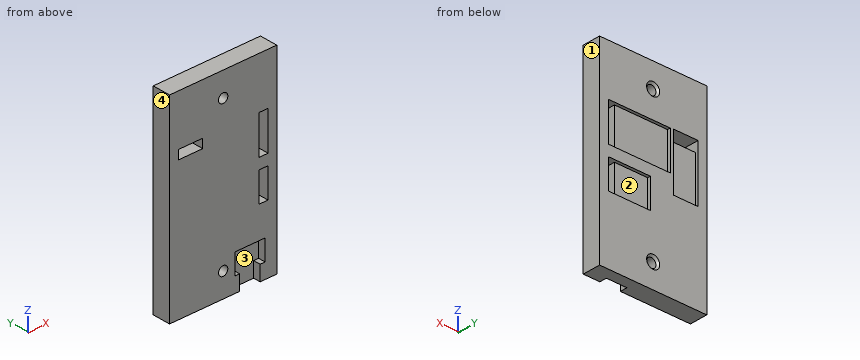
Autodesk Inventor part; units mm, degrees
ref_plane "작업 평면1" through (0, 10, 0) normal (0, 1, 0) x (1, 0, 0)
ref_plane "작업 평면2" through (0, 10, 0) normal (0, 1, 0) x (1, 0, 0)
ref_plane "작업 평면3" through (57.9435, 10, -25.2204) normal (0, 0, 1) x (1, 0, 0)
ref_plane "작업 평면1" through (0, 10, 0) normal (0, 1, 0) x (1, 0, 0)
sketch "스케치3" plane through (0, 10, 0) normal (0, 1, 0) x (1, 0, 0)
  line L0 (108.4435, 113.2704) -> (97.4435, 113.2704)
  line L1 (97.4435, 113.2704) -> (97.4435, 121.7204)
  line L2 (97.4435, 121.7204) -> (108.4435, 121.7204)
  line L3 (108.4435, 121.7204) -> (108.4435, 113.2704)
  line L4 (117.9435, 121.7204) -> (57.9435, 121.7204)
  line L5 (57.9435, 121.7204) -> (57.9435, 11.7204)
  line L6 (117.9435, 11.7204) -> (117.9435, 121.7204)
  line L7 (57.9435, 11.7204) -> (117.9435, 11.7204)
  line L8 (113.0685, 67.6907) -> (89.4185, 67.6907)
  line L9 (89.4185, 67.6907) -> (89.4185, 84.1907)
  line L10 (89.4185, 84.1907) -> (113.0685, 84.1907)
  line L11 (113.0685, 84.1907) -> (113.0685, 67.6907)
  line L12 (113.0684, 40.1407) -> (108.0685, 40.1407)
  line L13 (108.0685, 67.6907) -> (113.0685, 67.6907)
  line L14 (113.0684, 61.6907) -> (113.0684, 40.1407)
  line L15 (113.0685, 67.6907) -> (108.0685, 67.6907)
  line L16 (108.0685, 67.6907) -> (108.0685, 84.1907)
  line L17 (108.0685, 84.1907) -> (113.0685, 84.1907)
  line L18 (113.0685, 84.1907) -> (113.0685, 67.6907)
  line L19 (76.5185, 39.8907) -> (62.8185, 39.8907)
  line L20 (62.8185, 39.8907) -> (62.8185, 44.8907)
  line L21 (62.8185, 44.8907) -> (76.5185, 44.8907)
  line L22 (76.5185, 44.8907) -> (76.5185, 39.8907)
  line L23 (113.0684, 61.6907) -> (78.3675, 61.6907)
  circle A0 centre (87.9435, 25.2204) radius 2.6
  circle A1 centre (87.9435, 108.2204) radius 2.6
  line L24 (78.3675, 40.1407) -> (113.0684, 40.1407)
  line L25 (78.3675, 40.1407) -> (78.3675, 61.6907)
  line L26 (76.5185, 39.8907) -> (76.5185, 71.6407)
  line L27 (62.8185, 39.8907) -> (62.8185, 71.6407)
  line L28 (76.5185, 71.6407) -> (62.8185, 71.6407)
  line L29 (108.0685, 61.6907) -> (108.0685, 40.1407)
  point P0 (0, 0)
  dimension "d8" = 9.5
  dimension "d46" = 5.2
  dimension "d47" = 5.2
extrude "돌출2" add sketch "스케치3" against normal blind 10 contours L3 L4 L6 L7 L5 L1 L0 | L0 L1 L2 L3 | L8 L16 L10 L11 | L8 L9 L10 L16 | L12 L29 L23 L14 | L24 L25 L23 L29 | L19 L20 L21 L22 | L21 L27 L28 L26 | A0 | A1
sketch "스케치4" plane through (0, 10, 0) normal (0, 1, 0) x (1, 0, 0)
  point P0 (0, 0)
sketch "스케치5" plane through (117.9435, 10, -121.7204) normal (0, 0, -1) x (-1, 0, 0)
  point P0 (117.9435, -10)
extrude "돌출5" cut sketch "스케치3" against normal through all contours L0 L1 L2 L3
sketch "스케치6" plane through (0, 0, 0) normal (0, -1, 0) x (1, 0, 0)
  line L0 (57.9435, -121.7204) -> (97.4435, -121.7204)
  line L1 (97.4435, -121.7204) -> (57.9435, -121.7204)
  line L2 (113.0685, -71.6204) -> (108.0685, -71.6204)
  line L3 (113.0685, -80.2704) -> (113.0685, -71.6204)
  line L4 (78.3685, -80.2704) -> (113.0685, -80.2704)
  line L5 (78.3685, -58.4704) -> (78.3685, -80.2704)
  line L6 (113.0685, -58.4704) -> (78.3685, -58.4704)
  line L7 (113.0685, -67.1204) -> (113.0685, -58.4704)
  line L8 (108.0685, -67.1204) -> (113.0685, -67.1204)
  line L9 (108.0685, -71.6204) -> (108.0685, -67.1204)
  line L10 (117.9435, -121.7204) -> (108.4435, -121.7204)
  line L11 (111.4435, -108.7204) -> (94.443, -108.7204)
  line L12 (111.4435, -108.7204) -> (111.4435, -113.2704)
  line L13 (94.443, -108.7204) -> (94.443, -113.2704)
  line L14 (111.4435, -113.2704) -> (94.443, -113.2704)
  point P0 (0, 0)
sketch "스케치7" plane through (0, 0, 0) normal (0, -1, 0) x (1, 0, 0)
  point P0 (0, 0)
sketch "스케치8" plane through (0, 0, 0) normal (0, -1, 0) x (1, 0, 0)
  point P0 (0, 0)
extrude "돌출6" cut sketch "스케치6" against normal blind 4 contours L12 L14 L13 L11
extrude "돌출7" add sketch "스케치3" against normal blind 6 contours L0 L1 L2 L3
sketch "스케치9" plane through (0, 0, 0) normal (0, -1, 0) x (1, 0, 0)
  line L0 (111.4435, -108.7204) -> (111.4435, -113.2704)
  line L1 (111.4435, -108.7204) -> (111.4435, -101.7204)
  line L2 (111.4435, -101.7204) -> (94.443, -101.7204)
  line L3 (94.443, -113.2704) -> (94.443, -108.7204)
  line L4 (94.443, -101.7204) -> (94.443, -108.7204)
  line L5 (94.443, -108.7204) -> (111.4435, -108.7204)
  line L6 (111.4435, -108.7204) -> (94.443, -108.7204)
  point P0 (0, 0)
  dimension "d25" = 7
extrude "돌출8" cut sketch "스케치9" against normal blind 4
sketch "스케치10" plane through (0, 10, 0) normal (0, 1, 0) x (1, 0, 0)
  circle A0 centre (87.9435, 25.2204) radius 3.85
  circle A1 centre (87.9435, 108.2204) radius 3.85
  point P0 (0, 0)
  dimension "d28" = 7.7
  dimension "d29" = 7.7
ref_plane "작업 평면2" through (0, 10, 0) normal (0, 1, 0) x (1, 0, 0)
sketch "스케치12" plane through (0, 10, 0) normal (0, 1, 0) x (1, 0, 0)
  point P0 (0, 0)
ref_plane "작업 평면3" through (57.9435, 10, -25.2204) normal (0, 0, 1) x (1, 0, 0)
sketch "스케치13" plane through (57.9435, 10, -25.2204) normal (0, 0, 1) x (1, 0, 0)
  line L0 (30, 0) -> (30, -4)
  line L1 (30, 0) -> (33.65, 0)
  line L2 (33.65, 0) -> (30, -4)
  point P0 (-57.9435, -10)
  point P1 (32.25, 0)
  dimension "d35" = 4
  dimension "d36" = 3.65
sketch "스케치14" plane through (57.9435, 10, -25.2204) normal (0, 0, 1) x (1, 0, 0)
  point P0 (-57.9435, -10)
revolve "회전2" cut sketch "스케치13" angle 360 about axis through (87.9435, 10, -25.2204) along (0, -1, 0)
ref_plane "작업 평면4" through (57.9435, 10, -66.7204) normal (0, 0, 1) x (1, 0, 0)
mirror "미러1" about plane through (57.9435, 10, -66.7204) normal (0, 0, 1) of "회전2"
sketch "스케치15" plane through (0, 0, 0) normal (0, -1, 0) x (1, 0, 0)
  line L0 (108.6612, -121.7204) -> (97.1612, -121.7204)
  line L1 (97.1612, -121.7204) -> (97.1612, -113.2704)
  line L2 (108.6612, -121.7204) -> (108.6612, -113.2704)
  line L3 (97.1612, -113.2704) -> (108.6612, -113.2704)
  line L4 (97.4435, -113.2704) -> (94.443, -113.2704)
  point P0 (0, 0)
extrude "돌출9" cut sketch "스케치15" against normal blind 4
extrude "돌출11" cut sketch "스케치3" against normal through all contours A0 | A1
extrude "돌출12" cut sketch "스케치3" against normal through all contours L8 L16 L10 L11 | L12 L29 L23 L14 | L19 L20 L21 L22
extrude "돌출13" cut sketch "스케치3" against normal blind 1.7 contours L8 L9 L10 L16 | L24 L25 L23 L29 | L21 L27 L28 L26
properties part number "1구버전"
Work out the finished part from the listing and answer in its coordinate system (mm). Face numbers are marked on the shaded views. A direction names the side the tool comes from. Coordinates: 2 decimals unless noted, no trailing zeros. Order: outer loops, then holes, each group sorted by start corner. A loop starts at its lowest first (then second) coordinate and runs counter-clockwise, first axis right, second up. Notation, with made-up numbers: (33.5, 16.25) - (52.5, 16.25) arc R14 cw to (52.5, 22.25) - close; hole circle Ø3 at (61.5, 6). An arc over 180 degrees is marked (long way). Put each result on its own line as item: value. Start each with the question number.
1) Find section C-C (x = 107). Give the vertices of the cut face in (y, z), plus the area to 3 significant figures.
2) Find section B-B (y = 5.75). Give the vertices of the cut face in (x, z), plus the area to 3 significant figures.
3) Find the intervals of material crossed by line 1 (Z direction, x = 109, y = 6.5); line 2 (X direction, y = 9.75, z = -56.5); line 3 (Z direction, x = 111, y = 0.5), in increasing order. Write a range as from..to.
4) Find section A-A (x = 73). Give the vertices of the cut face in (y, z), plus the area to 3 significant figures.
5) Flat-ended cylindrical pins translate along their axes: pin 1 (11 mm diameter, centred on x = 70.5, z = -59, fed in from +Y); pin 2 (3 mm diameter, centred on x = 106.5, y = 1.5, fed in from -Z). Find the tip coordinate at first contact, or state that the pin passes through.
6) Find section D-D (x = 79.5). Give the vertices of the cut face in (y, z), plus the area to 3 significant figures.
7) For the marked faces 1 and 2, determine the directions among +Z, -Z, +X, -X, +Y, -Y from which every point of the face is accessible in a straight line to the end or side of a thin tool.
8) For a pull along Z with two mould halves and no side action, classify the marked faces 3 and 4 as released by +Z, released by -Z, zero draft, split by the parting line, or undercut.
Results list:
1. outline: (0, -101.72) - (4, -101.72) - (4, -121.72) - (10, -121.72) - (10, -84.19) - (8.3, -84.19) - (8.3, -67.69) - (10, -67.69) - (10, -61.69) - (8.3, -61.69) - (8.3, -40.14) - (10, -40.14) - (10, -11.72) - (0, -11.72) - close
1. area: 955 mm^2
2. outline: (57.94, -121.72) - (117.94, -121.72) - (117.94, -11.72) - (57.94, -11.72) - close; hole (62.82, -44.89) - (76.52, -44.89) - (76.52, -39.89) - (62.82, -39.89) - close; hole circle Ø5.2 at (87.94, -108.22); hole circle Ø5.2 at (87.94, -25.22); hole (108.07, -84.19) - (113.07, -84.19) - (113.07, -67.69) - (108.07, -67.69) - close; hole (108.07, -61.69) - (113.07, -61.69) - (113.07, -40.14) - (108.07, -40.14) - close
2. area: 6,300 mm^2
3. line 1: z = -121.72..-84.19, -67.69..-61.69, -40.14..-11.72
3. line 2: x = 57.94..62.82, 76.52..78.37, 113.07..117.94
3. line 3: z = -121.72..-113.27, -101.72..-84.19, -67.69..-61.69, -40.14..-11.72
4. outline: (0, -121.72) - (10, -121.72) - (10, -71.64) - (8.3, -71.64) - (8.3, -44.89) - (0, -44.89) - close; (0, -39.89) - (10, -39.89) - (10, -11.72) - (0, -11.72) - close
4. area: 1,000 mm^2
5. pin 1: stops at y = 8.3
5. pin 2: stops at z = -101.72
6. outline: (0, -121.72) - (10, -121.72) - (10, -61.69) - (8.3, -61.69) - (8.3, -40.14) - (10, -40.14) - (10, -11.72) - (0, -11.72) - close
6. area: 1,060 mm^2
7. face 1: +Z, -Z, +X, +Y, -Y
7. face 2: +Y
8. face 3: undercut
8. face 4: zero draft
